Source: CAD feature listing. Evaluate the final solid. Frame: model axes, mm. A direction names the side the tool comes from. Give positions to 0.01 mm unless a question says otherwise; leave off trailing zeros. Order: outer loops, then holes, each group sorted by start corner. A loop starts at its lowest first (then second) coordinate and runs counter-clockwise, first axis right, second up.
```python
from build123d import *

# Parameters (mm, degrees)
SKETCH1_R           = 1.5
BOSS_EXTRUDE1_DEPTH = 5
SKETCH2_R           = 3.5
CUT_EXTRUDE1_DEPTH  = 1
CUT_EXTRUDE2_DEPTH  = 3.9


with BuildPart() as part:
    # Sketch1 → Boss-Extrude1 (new, symmetric)
    with BuildSketch(Plane.XY):
        with BuildLine():
            ThreePointArc((-101.197826064, -28), (-105, 0), (-101.197826064, 28))
            ThreePointArc((-101.197826064, 28), (-106.426242211, 37.228416147), (-115.654658358, 32))
            ThreePointArc((-115.654658358, 32), (-120, 0), (-115.654658358, -32))
            ThreePointArc((-115.654658358, -32), (-106.426242211, -37.228416147), (-101.197826064, -28))
        make_face()
        with Locations((-108.426242211, -30)):
            Circle(SKETCH1_R, mode=Mode.SUBTRACT)
        with Locations((-108.426242211, 0)):
            Circle(SKETCH1_R, mode=Mode.SUBTRACT)
        with Locations((-108.426242211, 30)):
            Circle(SKETCH1_R, mode=Mode.SUBTRACT)
    extrude(amount=BOSS_EXTRUDE1_DEPTH, both=True)

    # Sketch2 → Cut-Extrude1 (cut)
    with BuildSketch(Plane.XY.offset(5)):
        with BuildLine():
            ThreePointArc((-103.125403703, 28.533333333), (-106.959575544, 35.300838508), (-113.727080719, 31.466666667))
            ThreePointArc((-113.727080719, 31.466666667), (-118, 0), (-113.727080719, -31.466666667))
            ThreePointArc((-113.727080719, -31.466666667), (-106.959575544, -35.300838508), (-103.125403703, -28.533333333))
            ThreePointArc((-103.125403703, -28.533333333), (-105.801637311, -15.969143446), (-106.952890403, -3.174781008))
            ThreePointArc((-106.952890403, -3.174781008), (-111.926242211, 0), (-106.952890403, 3.174781008))
            ThreePointArc((-106.952890403, 3.174781008), (-105.801637311, 15.969143446), (-103.125403703, 28.533333333))
        make_face()
        with Locations((-108.426242211, -30)):
            Circle(SKETCH2_R, mode=Mode.SUBTRACT)
        with Locations((-108.426242211, 30)):
            Circle(SKETCH2_R, mode=Mode.SUBTRACT)
    extrude(amount=-CUT_EXTRUDE1_DEPTH, mode=Mode.SUBTRACT)

    # Sketch3 → Cut-Extrude2 (cut, symmetric)
    with BuildSketch(Plane.XY):
        with BuildLine():
            ThreePointArc((-113.727080719, 31.466666667), (-111.610121749, 38.303795152), (-109.082537558, 45))
            Line((-109.082537558, 45), (-139.082537558, 45))
            Line((-139.082537558, 45), (-139.082537558, -45))
            Line((-139.082537558, -45), (-109.082537558, -45))
            ThreePointArc((-109.082537558, -45), (-111.610121749, -38.303795152), (-113.727080719, -31.466666667))
            ThreePointArc((-113.727080719, -31.466666667), (-118, 0), (-113.727080719, 31.466666667))
        make_face()
    extrude(amount=CUT_EXTRUDE2_DEPTH, both=True, mode=Mode.SUBTRACT)


solid = part.part
```
1) Section query A-A, the plane y = -30. Return the cut outline in (x, z), and give its area (3 significant figures).
Report:
outline: (-116.19, -5) - (-109.93, -5) - (-109.93, 5) - (-111.93, 5) - (-111.93, 4) - (-114.12, 4) - (-114.12, 5) - (-116.19, 5) - (-116.19, 3.9) - (-114.12, 3.9) - (-114.12, -3.9) - (-116.19, -3.9) - close; (-106.93, -5) - (-100.93, -5) - (-100.93, 5) - (-102.93, 5) - (-102.93, 4) - (-104.93, 4) - (-104.93, 5) - (-106.93, 5) - close
area: 102 mm2
2) Material intervals for L1, parallel to Z at x = -117.5, y = -16; L2, parallel to Y at x = -107.5, z = 1.5; L3, parallel to Y at x = -108, z = 2.5, sorted ascending.
Report:
L1: z = -5 to -3.9, 3.9 to 5
L2: y = -37.44 to -31.18, -28.82 to -1.18, 1.18 to 28.82, 31.18 to 37.44
L3: y = -37.49 to -31.44, -28.56 to -1.44, 1.44 to 28.56, 31.44 to 37.49
3) Section query D-D, the plane y = -19.5. Return the cut outline in (x, z).
Report:
outline: (-118.41, -5) - (-103.17, -5) - (-103.17, 5) - (-105.21, 5) - (-105.21, 4) - (-116.38, 4) - (-116.38, 5) - (-118.41, 5) - (-118.41, 3.9) - (-116.38, 3.9) - (-116.38, -3.9) - (-118.41, -3.9) - close
4) Pin query (flat end, axial travel): pin 1 (2.5 mm diameter, centred on x = -108.43, y = -30, fed in from -Z); pin 2 (1 mm diameter, centred on y = -6.5, z = 2, fed in from -X); pin 3 (5 mm diameter, centred on x = -110, y = 21, fed in from +Z); pin 4 (1 mm diameter, centred on y = -23.5, z = 2, fed in from +X). Return the tip coordinate at first contact, or that it passes through.
Report:
pin 1: passes through
pin 2: stops at x = -117.85
pin 3: stops at z = 4
pin 4: stops at x = -102.22
5) Section query B-B, the plane z = 1.5. Return the cut outline in (x, y), and give its area (3 significant figures).
Report:
outline: (-112.22, -36.47) arc R7.5 ccw to (-101.2, -28) arc R105 cw to (-101.2, 28) arc R7.5 ccw to (-112.22, 36.47) arc R118 ccw to start; hole circle Ø3 at (-108.43, -30); hole circle Ø3 at (-108.43, 0); hole circle Ø3 at (-108.43, 30)
area: 924 mm2
6) Section query C-C, the plane x = -108.25. Count the separate pieces of the cut face and the enclosed holes in it, and give its area (3 significant figures).
Report:
separate pieces: 4
enclosed holes: 0
area: 611 mm2
7) Reachability of faces 1 (the cylindrical face through (-104.21, -36.203, 0.07)), 2 (the cylindrical face through (-107.076, -35.332, 4.507)), 3 (the flat face through (-118.4, 0.2, -3.9)) from +Z, -Z, +X, -X, +Y, -Y: full face, straight path, thin tool, end or side. Return the list, or none.
Report:
face 1: +Z, -Z
face 2: +Z
face 3: -X
8) Draft query along X for faces 4 (the flat face through (-108, 28, 5)), 5 (the cylindrical face through (-106.996, 30.451, -0.07)), 6 (the cylindrical face through (-103.94, 36.01, 0.07)). Return one class per face: +X half, -X half, draft (parallel to the pull), parting line (faces both ways), or undercut.
Report:
face 4: draft
face 5: undercut
face 6: parting line
